Drawing for the job (mm, zero at the part's lowest x, y, z). A direction names the side the tool comes from. Give positions to 0.01 mm unless a question says otherwise; leave off trailing zeros. Order: outer loops, then holes, each group sorted by start corner. A loop starts at its lowest first (then second) coordinate and runs counter-clockwise, first axis right, second up. Notation, with made-up numbers: (52, 61) - (63, 61) arc R19 cw to (63, 90) - close; hole circle Ø5 at (-13, 24). An arc over 180 degrees is marked (long way). Use a Markdown table: item, result.
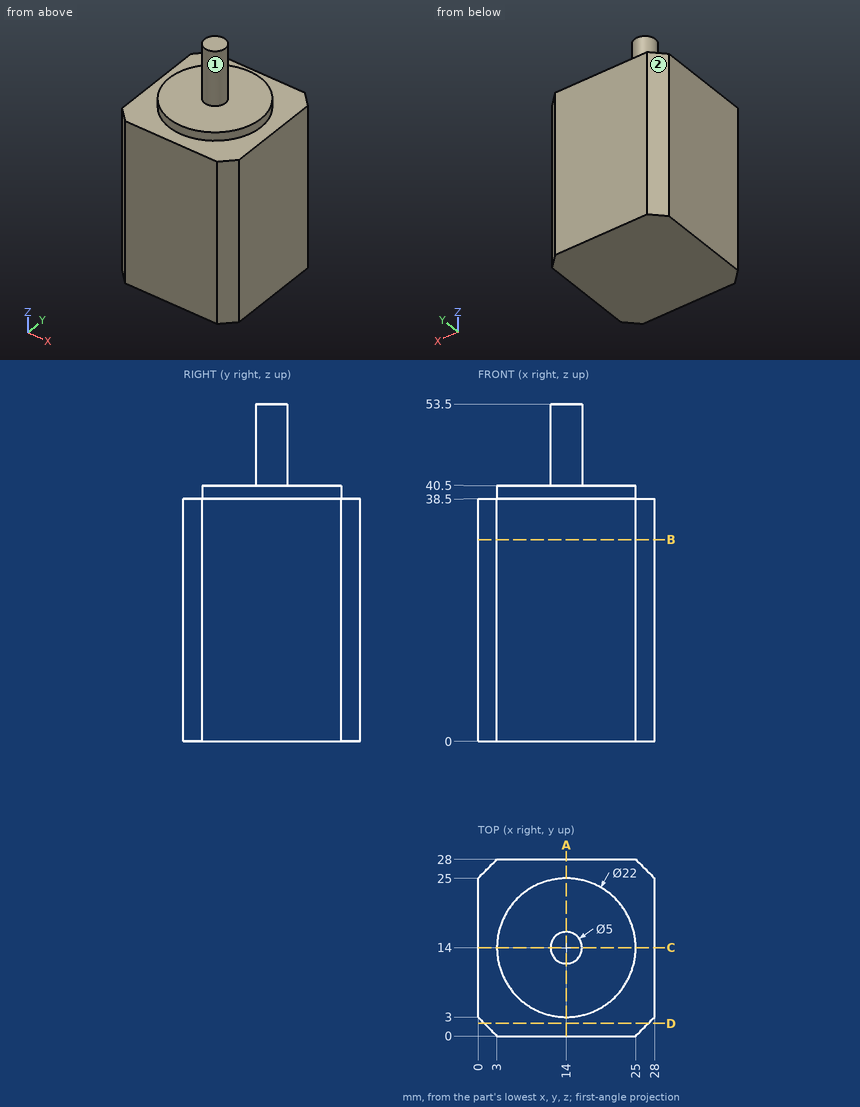
1) Slice it at A-A (x = 14). Write the cut outline in (y, z), and give its area (3 significant figures).
Computed:
| item | result |
|---|---|
| outline | (0, 0) - (28, 0) - (28, 38.5) - (25, 38.5) - (25, 40.5) - (16.5, 40.5) - (16.5, 53.5) - (11.5, 53.5) - (11.5, 40.5) - (3, 40.5) - (3, 38.5) - (0, 38.5) - close |
| area | 1,190 mm² |
2) Slice it at D-D (y = 2). Write the cut outline in (x, z), and give its area (3 significant figures).
Computed:
| item | result |
|---|---|
| outline | (1, 0) - (27, 0) - (27, 38.5) - (1, 38.5) - close |
| area | 1,000 mm² |
3) Wall check: line 1 (Z direction, x = 13.5, y = 18.5); line 2 (Z direction, x = 26.25, y = 3); line 3 (Y direction, x = 26.5, z = 20.5). Give the ranges that are in metal, low to high. Write a range as from..to.
Computed:
| item | result |
|---|---|
| line 1 | z = 0..40.5 |
| line 2 | z = 0..38.5 |
| line 3 | y = 1.5..26.5 |
4) Tool access for the marked faces 1 and 2: list every direction of +Z, -Z, +X, -X, +Y, -Y with a clear straight run to the whole face (end or side of a thin tool).
Computed:
| item | result |
|---|---|
| face 1 | +Z |
| face 2 | +Z, -Z, -X, +Y |
5) Slice it at B-B (z = 32). Write the cut outline in (x, y), and give its area (3 significant figures).
Computed:
| item | result |
|---|---|
| outline | (0, 3) - (3, 0) - (25, 0) - (28, 3) - (28, 25) - (25, 28) - (3, 28) - (0, 25) - close |
| area | 766 mm² |
